```python
from build123d import *

# Parameters (mm, degrees)
SKETCH1_R                = 25.4
HUB_MAIN_DEPTH           = 12.7
SKETCH2_R                = 3.175
HUB_BOLT_HOLES_DEPTH     = 13.7
CIRPATTERN1_COUNT        = 3
LEG_DEPTH                = 12.7
FILLET1_R                = 2.54
CIRPATTERN2_COUNT        = 5
FILLET1_OF_CIRPATTERN2_R = 2.54


with BuildPart() as part:
    # Sketch1 → Hub main (new body)
    with BuildSketch(Plane.XY):
        Circle(SKETCH1_R)
    extrude(amount=HUB_MAIN_DEPTH)

    # Sketch2 → Hub bolt holes (cut, through all)
    with BuildSketch(Plane.XY.offset(12.7)):
        with Locations((0, 15.875)):
            Circle(SKETCH2_R)
    hub_bolt_holes = extrude(amount=-HUB_BOLT_HOLES_DEPTH, mode=Mode.SUBTRACT)

    # CirPattern1: Hub bolt holes ×3 about axis
    cirpattern1_axis = Axis((0, -0.251984127, 0), (0, 0, 1))
    for i in range(1, CIRPATTERN1_COUNT):
        add(hub_bolt_holes.rotate(cirpattern1_axis, i * 360 / CIRPATTERN1_COUNT), mode=Mode.SUBTRACT)

    # Sketch4 → leg (add)
    with BuildSketch(Plane.XY.offset(12.7)):
        with BuildLine():
            Line((24.593444248, 6.35), (44.45, 6.35))
            Line((44.45, 6.35), (62.426544532, -11.626544532))
            ThreePointArc((62.426544532, -11.626544532), (61.641094588, -15.252064058), (60.645274989, -18.82553111))
            Line((60.645274989, -18.82553111), (41.819743879, 0))
            Line((41.819743879, 0), (25.4, 0))
            ThreePointArc((25.4, 0), (25.197554285, 3.200509029), (24.593444248, 6.35))
        make_face()
    leg = extrude(amount=-LEG_DEPTH)

    # Fillet1
    fillet1_edges = [part.edges().sort_by_distance(p)[0] for p in [
        (41.819743879, 0, 6.35),
        (44.45, 6.35, 6.35),
        (62.426544532, -11.626544532, 6.35),
        (60.645274989, -18.82553111, 6.35),
    ]]
    fillet(fillet1_edges, radius=FILLET1_R)

    # CirPattern2: leg ×5 about axis
    cirpattern2_axis = Axis((0, 0, 0), (0, 0, 1))
    for i in range(1, CIRPATTERN2_COUNT):
        add(leg.rotate(cirpattern2_axis, i * 360 / CIRPATTERN2_COUNT))

    # Fillet1 of CirPattern2
    fillet1_of_cirpattern2_edges = [part.edges().sort_by_distance(p)[0] for p in [
        (12.923011559, 39.772939926, 6.35),
        (7.696596521, 44.236720064, 6.35),
        (30.3483641, 55.778372121, 6.35),
        (36.644564635, 51.859674919, 6.35),
        (-33.832883498, 24.581028707, 6.35),
        (-39.693241752, 20.98979655, 6.35),
        (-43.670224016, 46.09947434, 6.35),
        (-37.997688541, 50.876572855, 6.35),
        (-33.832883498, -24.581028707, 6.35),
        (-32.228369048, -31.264312379, 6.35),
        (-57.338046838, -27.287330115, 6.35),
        (-60.128427647, -20.416223664, 6.35),
        (12.923011559, -39.772939926, 6.35),
        (19.775014278, -40.312204235, 6.35),
        (8.233362221, -62.963971814, 6.35),
        (0.836276565, -63.494493001, 6.35),
    ]]
    fillet(fillet1_of_cirpattern2_edges, radius=FILLET1_OF_CIRPATTERN2_R)


solid = part.part
```
Part model, mm, in its own coordinate system. A direction names the side the tool comes from. Coordinates: 2 decimals unless noted, no trailing zeros. Write each loop counter-clockwise with the first axis right and the second up, starting at its lowest first coordinate (ties: lowest second). Pieces come first, ordered by that corner, then holes.
Item 1: Slice it at D-D (z = 6.5). Count the separate pieces of the cut face and the enclosed holes in it, and give its area (3 significant figures).
Item 2: Slice it at B-B (x = 15.5). Write the cut outline in (y, z).
Item 3: Probe line 1 (X direction, y = 37, z = 1); line 2 (Y direction, x = -8.5, z = 4); line 3 (Y direction, x = -32, z = 10). List the from-to ranges inside material, lowest first.
Item 4: Mould opens along Y. For faces 1 (the face through (-31.13, 14.77, 6.44)), 2 (the face through (50.16, -8.34, 6.44)), 3 (the face through (-38.984, 48.554, 6.261)) say: released by +Y, released by -Y, zero draft, split by the parting line, or undercut.
Item 5: Which spindle directions (+Z, -Z, +X, -X, +Y, -Y) get a long thin tool onto all of the face, cutting with end or side? Do faces 4 (the face through (34, 6.35, 6)), 5 (the face through (-35.678, 36.233, 6.439)), 6 (the face through (-4.92, -24.92, 6.26)). Say none if no direction does.
Item 6: Pin check, flat tips, straight feed: pin 1 (6 mm diameter, centred on y = -29.5, z = 2.5, fed in from -X); pin 2 (5 mm diameter, centred on x = 24.5, z = 2.5, fed in from +Y); pin 3 (4 mm diameter, centred on x = -28.5, z = 3, fed in from -Y); pin 4 (10 mm diameter, centred on x = -13.97, y = -8.32, fed in from -Z). Stop position of each tip, or through.
Item 7: Slice it at A-A (x = 0). Write the cut outline in (y, z).
Item 8: Slice it at C-C (x = -22). Write the cut outline in (y, z).
Results found:
1. separate pieces: 1
1. enclosed holes: 3
1. area: 3,310 mm2
2. outline: (-48.7, 0) - (-27.16, 0) - (-27.16, 12.7) - (-48.7, 12.7) - close; (-20.12, 0) - (-11.1, 0) - (-11.1, 12.7) - (-20.12, 12.7) - close; (-5.54, 0) - (20.12, 0) - (20.12, 12.7) - (-5.54, 12.7) - close; (41.09, 0) - (48.21, 0) - (48.21, 12.7) - (41.09, 12.7) - close
3. line 1: x = -42.23 to -35.8, 5.35 to 12.02
3. line 2: y = -23.94 to 23.94
3. line 3: y = -30.98 to -23.25, 15.4 to 23.25
4. face 1: undercut
4. face 2: released by -Y
4. face 3: released by +Y
5. face 4: +Z, -Z, +X
5. face 5: +Z, -Z, +Y
5. face 6: +Z, -Z
6. pin 1: stops at x = -57.64
6. pin 2: stops at y = 54.07
6. pin 3: stops at y = -30.01
6. pin 4: stops at z = 0
7. outline: (-25.4, 0) - (12.7, 0) - (12.7, 12.7) - (-25.4, 12.7) - close; (19.05, 0) - (25.4, 0) - (25.4, 12.7) - (19.05, 12.7) - close
8. outline: (-23.83, 0) - (-15.98, 0) - (-15.98, 12.7) - (-23.83, 12.7) - close; (-12.69, 0) - (15.98, 0) - (15.98, 12.7) - (-12.69, 12.7) - close
